Input: part model. Units: mm. Frame: model coordinates. A direction names the side the tool comes from. Round coordinates to 2 decimals unless told otherwise and drop trailing zeros. Loops run counter-clockwise (first coordinate to the right, second up) from the corner with the lowest first, then second, coordinate; pieces in that order, holes last.
1) Ray query, line 1 along X through (y, z) = (11, -12); line 2 along Z through (x, y) = (-22, 2); line 3 along Y through (x, z) = (0.5, 15). Return the intervals inside material, ascending.
2) Section A-A, the plane y = 48. Return loops of the section in (x, z), and give its area (3 significant figures).
3) Draft query along Z for faces 3 (the face through (-1, 1, 30.111)), 4 (the face through (-7, 0, -7)), 5 (the face through (21.842, 1.521, -21.003)). Return one class per face: pulls with the +Z half, pulls with the -Z half, needs draft (parallel to the pull), parting line crosses it, or undercut.
4) Section B-B, the plane x = 26. Return loops of the section in (y, z), and give its area (3 significant figures).
5) Access query for faces 1 (the face through (-30.083, 1, 1)), 2 (the face through (16.166, 29.636, 0.112)). Directions: +Z, -Z, +X, -X, +Y, -Y. A direction counts if a zero-diameter tool reaches every point of the face in a straight line with its end or side. Return the directions, or none.
6) First-contact query: pin 1 (5 mm diameter, centred on x = 22.42, z = 22.61, fed in from +Y); pin 2 (6 mm diameter, centred on y = 16.5, z = -14, fed in from -X); pin 3 (3 mm diameter, centred on y = 29, z = 17.5, fed in from +X). Flat tips, straight axial feed; report the tip coordinate or a pass-through.
7) Section C-C, the plane z = 26.5. Return loops of the section in (x, y), and give its area (3 significant figures).
from build123d import *

# Parameters (mm, degrees)
SKETCH1_W                 = 60
SKETCH1_H                 = 60
SKETCH1_R                 = 8.884108342
SKETCH1_R_2               = 1.5
BOSS_EXTRUDE2_DEPTH       = 3
SKETCH2_R                 = 1.5
CUT_EXTRUDE1_DEPTH        = 10
BOSS_EXTRUDE3_OUTLINE_R   = 2.6
BOSS_EXTRUDE3_OUTLINE_R_2 = 4
BOSS_EXTRUDE3_DEPTH       = 53
FILLET1_R                 = 1
FILLET2_R                 = 1


# Read off the part's stored shape, not the designer's step: Boss-Extrude3
with BuildPart() as part:
    # Sketch1 → Boss-Extrude2 (new body)
    with BuildSketch(Plane(origin=(0, 0, 0), x_dir=(1, 0, 0), z_dir=(0, 1, 0))):
        with Locations((-0.083367938, -0.111157251)):
            Rectangle(SKETCH1_W, SKETCH1_H)
        with Locations(Location((-0.083367938, -0.111157251, 0), (0, 0, 270))):
            Circle(SKETCH1_R, mode=Mode.SUBTRACT)
        with Locations(Location((-10.515094807, -7.403555658, 0), (0, 0, 270))):
            Circle(SKETCH1_R_2, mode=Mode.SUBTRACT)
        with Locations(Location((7.209030469, -10.54288412, 0), (0, 0, 270))):
            Circle(SKETCH1_R_2, mode=Mode.SUBTRACT)
        with Locations(Location((10.348358931, 7.181241156, 0), (0, 0, 270))):
            Circle(SKETCH1_R_2, mode=Mode.SUBTRACT)
        with Locations(Location((-7.375766345, 10.320569618, 0), (0, 0, 270))):
            Circle(SKETCH1_R_2, mode=Mode.SUBTRACT)
    extrude(amount=BOSS_EXTRUDE2_DEPTH)

    # Sketch2 → Cut-Extrude1 (cut)
    with BuildSketch(Plane(origin=(0, 3, 0), x_dir=(1, 0, 0), z_dir=(0, 1, 0))):
        with Locations(Location((-22.583367938, 22.388842749, 0), (0, 0, 270))):
            Circle(SKETCH2_R)
        with Locations(Location((22.416632062, 22.388842749, 0), (0, 0, 270))):
            Circle(SKETCH2_R)
        with Locations(Location((22.416632062, -22.611157251, 0), (0, 0, 270))):
            Circle(SKETCH2_R)
        with Locations(Location((-22.5, -22.5, 0), (0, 0, 270))):
            Circle(SKETCH2_R)
    extrude(amount=-CUT_EXTRUDE1_DEPTH, mode=Mode.SUBTRACT)

    # Boss-Extrude3 outline → Boss-Extrude3 (add)
    # profile 1 of 3: a face of its own
    with BuildSketch(Plane(origin=(0, 3, 0), x_dir=(1, 0, 0), z_dir=(0, 1, 0))):
        with BuildLine():
            ThreePointArc((-8.871870842, 10.428603567), (-8.778562467, 10.85175983), (-8.568187528, 11.230587048))
            ThreePointArc((-8.568187528, 11.230587048), (-16.180054368, 13.654447968), (-8.871870842, 10.428603567))
        make_face()
        with Locations((-12.43926471, 12.237940737)):
            Circle(BOSS_EXTRUDE3_OUTLINE_R, mode=Mode.SUBTRACT)
    # profile 2 of 3: a face of its own
    with BuildSketch(Plane(origin=(0, 3, 0), x_dir=(1, 0, 0), z_dir=(0, 1, 0))):
        with Locations((-4.806777383, -16.774903612)):
            Circle(BOSS_EXTRUDE3_OUTLINE_R_2)
        with Locations((-4.806777383, -16.774903612)):
            Circle(BOSS_EXTRUDE3_OUTLINE_R, mode=Mode.SUBTRACT)
    # profile 3 of 3: a face of its own
    with BuildSketch(Plane(origin=(0, 3, 0), x_dir=(1, 0, 0), z_dir=(0, 1, 0))):
        with Locations((17.032817093, 3.792840871)):
            Circle(BOSS_EXTRUDE3_OUTLINE_R_2)
        with Locations((17.032817093, 3.792840871)):
            Circle(BOSS_EXTRUDE3_OUTLINE_R, mode=Mode.SUBTRACT)
    extrude(amount=BOSS_EXTRUDE3_DEPTH)

    # Fillet1
    # the kernel refuses this fillet: 1 mm, written as the material it adds along each edge
    with BuildSketch(Plane(origin=(-12.43926471, 3, -12.237940737), x_dir=(0.9363053197768356, 0, 0.3511870557944836), z_dir=(-0.3511870557944836, 0, 0.9363053197768356))) as fillet1_piece_1_section:
        with BuildLine():
            CenterArc((4 + FILLET1_R, FILLET1_R), FILLET1_R, 180, 90)
            Line((4, FILLET1_R), (4, 0))
            Line((4, 0), (4 + FILLET1_R, 0))
        make_face()
    fillet1_piece_1 = revolve(axis=Axis((-12.43926471, 3, -12.237940737), (0, 1, 0)), revolution_arc=359.64, mode=Mode.PRIVATE)
    fillet1_piece_1 = fillet1_piece_1 - Plane(origin=(-7.375766345, 3.279775491, -10.320569618), x_dir=(0, 0, 1), z_dir=(0, -1, 0)) * Cylinder(1.5, 21, mode=Mode.PRIVATE)
    add(fillet1_piece_1)

    # Fillet2
    fillet2_edges = [part.edges().sort_by_distance(p)[0] for p in [
        (-8.806777383, 3, 16.774903612),
        (-8.806777383, 56, 16.774903612),
        (13.032817093, 3, -3.792840871),
    ]]
    fillet(fillet2_edges, radius=FILLET2_R)


solid = part.part
Final values:
1. line 1: x = -16.43 to -15.03, -9.85 to -8.45
1. line 2: z = -29.89 to -23.77, -21.01 to 21.09, 23.91 to 30.11
1. line 3: y = 0 to 3
2. outline: (-8.87, -10.43) arc R4 ccw (long way) to (-8.57, -11.23) arc R1.5 cw to start; circle Ø8 at (-4.81, 16.77); circle Ø8 at (17.03, -3.79); hole circle Ø5.2 at (-12.44, -12.24); hole circle Ø5.2 at (-4.81, 16.77); hole circle Ø5.2 at (17.03, -3.79)
2. area: 87.0 mm2
3. face 3: pulls with the +Z half
3. face 4: needs draft
3. face 5: undercut
4. outline: (0, -29.89) - (3, -29.89) - (3, 30.11) - (0, 30.11) - close
4. area: 180 mm2
5. face 1: +Z, -Z, -X, +Y, -Y
5. face 2: +Y
6. pin 1: stops at y = 3
6. pin 2: stops at x = -16.44
6. pin 3: stops at x = -0.81
7. outline: (-30.08, 0) - (29.92, 0) - (29.92, 3) - (-30.08, 3) - close
7. area: 180 mm2
